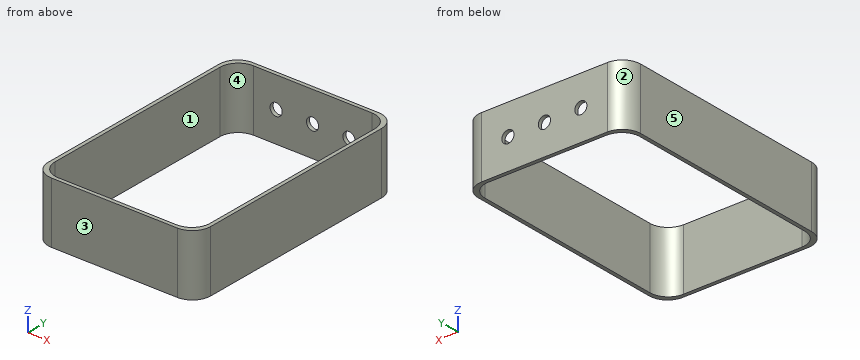
Autodesk Fusion 360 part; units mm, degrees
sketch "Sketch1" plane through (0, 0, 0) normal (0, 0, 1) x (1, 0, 0)
  line L0 (51.75, -99.5) -> (-51.75, -99.5)
  line L1 (-66.75, -84.5) -> (-66.75, 84.5)
  line L2 (-51.75, 99.5) -> (51.75, 99.5)
  line L3 (66.75, 84.5) -> (66.75, -84.5)
  line L4 (66.75, -99.5) -> (-66.75, 99.5) construction
  line L5 (-66.75, -99.5) -> (66.75, 99.5) construction
  line L6 (48.75, 96.5) -> (-48.75, 96.5)
  line L7 (-63.75, 81.5) -> (-63.75, -81.5)
  line L8 (-48.75, -96.5) -> (48.75, -96.5)
  line L9 (63.75, -81.5) -> (63.75, 81.5)
  line L10 (63.75, 96.5) -> (-63.75, -96.5) construction
  line L11 (-63.75, 96.5) -> (63.75, -96.5) construction
  arc A0 (-63.75, -81.5) -> (-48.75, -96.5) centre (-48.75, -81.5) ccw
  arc A1 (-66.75, -84.5) -> (-51.75, -99.5) centre (-51.75, -84.5) ccw
  arc A2 (48.75, -96.5) -> (63.75, -81.5) centre (48.75, -81.5) ccw
  arc A3 (51.75, -99.5) -> (66.75, -84.5) centre (51.75, -84.5) ccw
  arc A4 (63.75, 81.5) -> (48.75, 96.5) centre (48.75, 81.5) ccw
  arc A5 (66.75, 84.5) -> (51.75, 99.5) centre (51.75, 84.5) ccw
  arc A6 (-51.75, 99.5) -> (-66.75, 84.5) centre (-51.75, 84.5) ccw
  arc A7 (-48.75, 96.5) -> (-63.75, 81.5) centre (-48.75, 81.5) ccw
  dimension "d1" = 133.5
  dimension "d2" = 199
  dimension "d3" = 127.5
  dimension "d4" = 193
  dimension "d5" = 15
  dimension "d6" = 15
  dimension "d7" = 15
  dimension "d8" = 15
  dimension "d9" = 15
  dimension "d10" = 15
  dimension "d11" = 15
  dimension "d12" = 15
extrude "Extrude1" add sketch "Sketch1" along normal blind 10
extrude "Extrude2" add 1 faces at (65.75, -27.1667, 10) along direction (0, 0, 1) blind 10
extrude "Extrude3" add 1 faces at (65.75, -27.1667, 20) along direction (0, 0, 1) blind 30
sketch "Sketch2" plane through (0, 99.5, 0) normal (0, 1, 0) x (-1, 0, 0)
  line L0 (-51.75, 0) -> (51.75, 0)
  line L1 (51.75, 0) -> (51.75, 50)
  line L2 (51.75, 50) -> (-51.75, 50)
  line L3 (-51.75, 50) -> (-51.75, 0)
  circle A0 centre (0, 25) radius 5
  circle A1 centre (30, 25) radius 5
  circle A2 centre (-30, 25) radius 5
  dimension "d19" = 10
  dimension "d20" = 10
  dimension "d21" = 10
extrude "Extrude4" cut sketch "Sketch2" against normal blind 10 contours A0 | A1 | A2
Geometry check sheet. Reference: the model listing, model coordinates, mm. Face numbers are marked on the shaded views. A direction names the side the tool comes from. Coordinates: 2 decimals unless noted, no trailing zeros. Loops run counter-clockwise (first coordinate to the right, second up) from the corner with the lowest first, then second, coordinate; pieces in that order, holes last. Notation, with made-up numbers: (45.25, -22) -> (80.25, -22) arc R24 cw to (80.25, 3) -> close; hole circle Ø6 at (86, 36.5). An arc over 180 degrees is marked (long way). Put each result on its own line as item: value.
1) Release check for a two-part mould opening along Y. For the marked faces 3, 4 and 5 record: released by +Y, released by -Y, zero draft, split by the parting line, or undercut.
Result set:
face 3: released by -Y
face 4: undercut
face 5: zero draft
2) Cross-section at C-C on y = 7.5. Record the boundary of the cut face in (x, z), plus the area to 3 significant figures.
Result set:
outline: (-66.75, 0) -> (-63.75, 0) -> (-63.75, 50) -> (-66.75, 50) -> close; (63.75, 0) -> (66.75, 0) -> (66.75, 50) -> (63.75, 50) -> close
area: 300 mm^2
3) Cross-section at D-D on x = -17. Record the boundary of the cut face in (y, z).
Result set:
outline: (-99.5, 0) -> (-96.5, 0) -> (-96.5, 50) -> (-99.5, 50) -> close; (96.5, 0) -> (99.5, 0) -> (99.5, 50) -> (96.5, 50) -> close
4) Gauge pin test, flat end, axial feed: pin 1 Ø8 at (x, z) = (0, 25) entering from +Y. Record the tip position at first contact, or that the pin passes through.
Result set:
pin 1: stops at y = -96.5
5) Tool access check on the marked faces 1 and 2. Record the directions out of +Z, -Z, +X, -X, +Y, -Y that give a thin tool (end or side, any length) a straight path to the whole face; none if there is none.
Result set:
face 1: +Z, -Z
face 2: +Z, -Z, -X, +Y
6) Cross-section at A-A on z = 25. Record the boundary of the cut face in (x, y), plus the area to 3 significant figures.
Result set:
outline: (-66.75, -84.5) arc R15 ccw to (-51.75, -99.5) -> (51.75, -99.5) arc R15 ccw to (66.75, -84.5) -> (66.75, 84.5) arc R15 ccw to (51.75, 99.5) -> (35, 99.5) -> (35, 96.5) -> (48.75, 96.5) arc R15 cw to (63.75, 81.5) -> (63.75, -81.5) arc R15 cw to (48.75, -96.5) -> (-48.75, -96.5) arc R15 cw to (-63.75, -81.5) -> (-63.75, 81.5) arc R15 cw to (-48.75, 96.5) -> (-35, 96.5) -> (-35, 99.5) -> (-51.75, 99.5) arc R15 ccw to (-66.75, 84.5) -> close; (-25, 96.5) -> (-5, 96.5) -> (-5, 99.5) -> (-25, 99.5) -> close; (5, 96.5) -> (25, 96.5) -> (25, 99.5) -> (5, 99.5) -> close
area: 1,870 mm^2
7) Cross-section at B-B on x = 33. Record the boundary of the cut face in (y, z), plus the area to 3 significant figures.
Result set:
outline: (-99.5, 0) -> (-96.5, 0) -> (-96.5, 50) -> (-99.5, 50) -> close; (96.5, 0) -> (99.5, 0) -> (99.5, 21) -> (96.5, 21) -> close; (96.5, 29) -> (99.5, 29) -> (99.5, 50) -> (96.5, 50) -> close
area: 276 mm^2
8) Thickness scan on line 1 (Y direction, x = -6, z = 13); line 2 (Z direction, x = 0, y = 97.95); line 3 (X direction, y = 10.5, z = 35). Record the ranges inside material, lowest first.
Result set:
line 1: y = -99.5 to -96.5, 96.5 to 99.5
line 2: z = 0 to 20, 30 to 50
line 3: x = -66.75 to -63.75, 63.75 to 66.75
